from build123d import *

# Parameters (mm, degrees)
SKETCH2_R                    = 3.15
BASE_FLANGE1_DEPTH           = 3.175
EDGE_FLANGE1_STRIP_W         = 20.85
EDGE_FLANGE1_STRIP_H         = 3.175
EDGE_FLANGE1_STRIP_CUT_DEPTH = 37
EDGE_FLANGE1_DEPTH           = 37
SKETCH10_R                   = 3.15
CUT_EXTRUDE1_DEPTH           = 10


# Sheet-metal steps are written as plain solids
with BuildPart() as part:
    # Sketch2 → Base-Flange1 (new body)
    with BuildSketch(Plane(origin=(0, 0, 0), x_dir=(0, 0, -1), z_dir=(1, 0, 0))):
        with BuildLine():
            Line((48.551064785, 40.291218586), (48.551064785, 72.093066751))
            Line((48.551064785, 72.093066751), (14.602650648, 58.297559694))
            ThreePointArc((14.602650648, 58.297559694), (12.37556545, 56.443388888), (11.551064785, 53.665249851))
            Line((11.551064785, 53.665249851), (11.551064785, 40.291218586))
            Line((11.551064785, 40.291218586), (48.551064785, 40.291218586))
        make_face()
        with Locations((39.011220588, 57.194773579)):
            Circle(SKETCH2_R, mode=Mode.SUBTRACT)
        with Locations((20.490203266, 52.672523101)):
            Circle(SKETCH2_R, mode=Mode.SUBTRACT)
    extrude(amount=-BASE_FLANGE1_DEPTH)

    # Edge-Flange1 strip (across the edge) → Edge-Flange1 strip cut (cut)
    with BuildSketch(Plane(origin=(-3.175, 38.491218586, -48.551064785), x_dir=(0, 1, 0), z_dir=(0, 0, 1))):
        with Locations((-4.075, -1.5875)):
            Rectangle(EDGE_FLANGE1_STRIP_W, EDGE_FLANGE1_STRIP_H)
    extrude(amount=EDGE_FLANGE1_STRIP_CUT_DEPTH, mode=Mode.SUBTRACT)

    # Edge-Flange1 section (across the edge) → Edge-Flange1 (add)
    with BuildSketch(Plane(origin=(-3.175, 38.491218586, -48.551064785), x_dir=(0, 1, 0), z_dir=(0, 0, 1))):
        with BuildLine():
            Line((0, 3.175), (0, 12.825))
            Line((0, 12.825), (3.175, 12.825))
            Line((3.175, 12.825), (3.175, 3.175))
            ThreePointArc((3.175, 3.175), (4.10493597, 0.92993597), (6.35, 0))
            Line((6.35, 0), (6.35, -3.175))
            ThreePointArc((6.35, -3.175), (1.859871939, -1.315128061), (0, 3.175))
        make_face()
    extrude(amount=EDGE_FLANGE1_DEPTH)

    # Sketch10 → Cut-Extrude1 (cut)
    with BuildSketch(Plane(origin=(0, 41.666218586, 0), x_dir=(1, 0, 0), z_dir=(0, 1, 0))):
        with Locations(Location((-11.175, 30.051064785, 0), (0, 0, 180))):
            Circle(SKETCH10_R)
    extrude(amount=-CUT_EXTRUDE1_DEPTH, mode=Mode.SUBTRACT)


solid = part.part
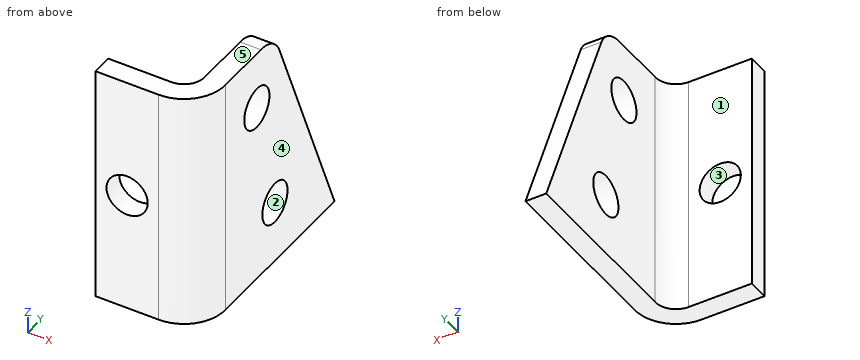
Can you work these out from the model? Positions are in its coordinate system, mm. Face numbers are marked on the shaded views. A direction names the side the tool comes from. Round coordinates to 2 decimals unless told otherwise and drop trailing zeros. Write each loop counter-clockwise with the first axis right and the second up, starting at its lowest first coordinate (ties: lowest second). Pieces come first, ordered by that corner, then holes. Notation, with made-up numbers: M -26.75,68 L 10.25,68 A27 ccw 10.25,86 Z; hole C -30,84 d2. An arc over 180 degrees is marked long. Use a Markdown table: item, result.
Item 1: For pin 1 Ø6 at (y, z) = (58.5, -22) entering from -X (3 decimals); pin 2 Ø5 at (x, z) = (-1.5, -19) entering from +Y; pin 3 Ø7.5 at (x, z) = (-9, -31.5) entering from +Y, each with a flat end and sliding along its axis, tell me the tip position at first contact or that it passes through.
Found:
| item | result |
|---|---|
| pin 1 | stops at x = -3.175 |
| pin 2 | stops at y = 61.1 |
| pin 3 | stops at y = 41.86 |
Item 2: I want a section at B-B (y = 52). List the corners of the cut face in (x, z) for me (3 decimals), and give its area (3 significant figures).
Found:
| item | result |
|---|---|
| outline | M -3.175,-48.551 L 0,-48.551 L 0,-23.568 L -3.175,-23.568 Z; M -3.175,-17.413 L 0,-17.413 L 0,-11.551 L -3.175,-11.551 Z |
| area | 97.9 mm2 |
Item 3: I want a section at D-D (z = -45). List the corners of the cut face in (x, y) for me (3 decimals), and give its area (3 significant figures).
Found:
| item | result |
|---|---|
| outline | M -16,38.491 L -6.35,38.491 A6.35 ccw 0,44.841 L 0,70.65 L -3.175,70.65 L -3.175,44.841 A3.175 cw -6.35,41.666 L -16,41.666 Z |
| area | 136 mm2 |
Item 4: If I drill on line 1 along X through (y, z) = (58.5, -19) (3 decimals); line 2 along Y through (x, z) = (-12.25, -15.5); line 3 along Z through (x, y) = (-1.5, 60.5), over which ranges is the centre line in solid material (lowest first)? Write a range as [from, to].
Found:
| item | result |
|---|---|
| line 1 | x = [-3.175, 0] |
| line 2 | y = [38.49, 41.67] |
| line 3 | z = [-48.55, -20.02] |
Item 5: We'd pull the mould along Z, two halves only. Please class the marked faces 3, 4 and 5: released by +Z, released by -Z, zero draft, split by the parting line, or undercut.
Found:
| item | result |
|---|---|
| face 3 | undercut |
| face 4 | zero draft |
| face 5 | released by +Z |
Item 6: Which directions (+Z, -Z, +X, -X, +Y, -Y) give clear straight access to the entire face, cutting with the end or side of a thin tool? Please do the marked faces 1 and 2.
Found:
| item | result |
|---|---|
| face 1 | +Z, -Z, -X, +Y |
| face 2 | +X, -X |
Item 7: I want a section at A-A (z = -21.5). List the corners of the cut face in (x, y) for me (3 decimals).
Found:
| item | result |
|---|---|
| outline | M -16,38.491 L -6.35,38.491 A6.35 ccw 0,44.841 L 0,49.689 L -3.175,49.689 L -3.175,44.841 A3.175 cw -6.35,41.666 L -16,41.666 Z; M -3.175,55.656 L 0,55.656 L 0,61.1 L -3.175,61.1 Z |
Item 8: I want a section at C-C (x = -12.5). List the corners of the cut face in (y, z) for me, and give its area (3 significant figures).
Found:
| item | result |
|---|---|
| outline | M 38.49,-48.55 L 41.67,-48.55 L 41.67,-32.91 L 38.49,-32.91 Z; M 38.49,-27.19 L 41.67,-27.19 L 41.67,-11.55 L 38.49,-11.55 Z |
| area | 99.3 mm2 |
